Here's how the part is built. I have some questions about the finished solid (model axes, mm). A direction names the side the tool comes from. Give positions to 0.01 mm unless a question says otherwise; leave off trailing zeros. Loops run counter-clockwise (first coordinate to the right, second up) from the corner with the lowest first, then second, coordinate; pieces in that order, holes last. Notation, with made-up numbers: (56, 9.5) - (66, 9.5) arc R22 ccw to (66, 21.5) - close; hole circle Ø8 at (-10, 7.25). An arc over 180 degrees is marked (long way). Use a Markdown table: item, result.
from build123d import *

# Parameters (mm, degrees)
F1_R   = 30
F1_R_2 = 29


with BuildPart() as f2:
    # F2: sweep along a path in F0
    with BuildLine(Plane.YZ) as f2_path:
        Line((0, 0), (0, 455))
        ThreePointArc((0, 455), (13.180195, 486.819805), (45, 500))
        Line((45, 500), (255, 500))
        ThreePointArc((255, 500), (286.819805, 513.180195), (300, 545))
        Line((300, 545), (300, 650))
    # F1 (on Top) → F2 (sweep)
    with BuildSketch(Plane.XY):
        Circle(F1_R)
        Circle(F1_R_2, mode=Mode.SUBTRACT)
    sweep(path=f2_path.line)


solid = f2.part
(1) Will these pins go through, and if not, where does the flat tip stop? pin 1 (8 mm diameter, centred on x = 11, z = 99.5, fed in from +Y); pin 2 (1 mm diameter, centred on x = -3.5, z = 150, fed in from -Y); pin 3 (10 mm diameter, centred on x = -9.5, y = 114, fed in from +Z).
A:
| item | result |
|---|---|
| pin 1 | y = 29.17 |
| pin 2 | y = -29.85 |
| pin 3 | z = 529.66 |
(2) If I drill on line 1 (Y direction, x = 0, z = 611); line 2 (Z direction, x = -1, y = 242); line 3 (X direction, y = 300, z = 606.5), over which ranges is the centre line in solid material (lowest first)?
A:
| item | result |
|---|---|
| line 1 | 270 to 271, 329 to 330 |
| line 2 | 470.02 to 471.02, 528.98 to 529.98 |
| line 3 | -30 to -29, 29 to 30 |
(3) On a 3-axis mill with a long thin cutter (end or side, diameter ignored), from which of +Z, -Z, +X, -X, +Y, -Y can I reach the whole of each face in a straight line? I mean faces 1 (the face through (13.843, 273.385, 598.235)), 2 (the face through (13.38, -25.73, 230.68)), 3 (the face through (-16, 325, 650)). Say none if no direction works.
A:
| item | result |
|---|---|
| face 1 | +Z |
| face 2 | -Z |
| face 3 | +Z, +X, -X, +Y, -Y |
(4) We'd pull the mould along X, two halves only. Please class faces 4 (the face through (-29.97, 1.32, 230.68)), 5 (the face through (-6.29, 271.69, 598.24)), 6 (the face through (-16, 25, 0)): pulls with the +X half, pulls with the -X half, needs draft (parallel to the pull), parting line crosses it, or undercut.
A:
| item | result |
|---|---|
| face 4 | parting line crosses it |
| face 5 | undercut |
| face 6 | needs draft |
(5) Suppose I cut it at A-A on z = 225. Write out the boundary of the cut face in (x, y), plus the area to 3 significant figures.
A:
| item | result |
|---|---|
| outline | circle Ø60 at (0, 0); hole circle Ø58 at (0, 0) |
| area | 185 mm2 |
